Design review of the part shown in the three views and the two pictorial views. Dimensions are in mm from the part's minimum x, y and z. Round coordinates to 2 decimals unless told otherwise and drop trailing zeros. Write each loop counter-clockwise with the first axis right and the second up, starting at its lowest first coordinate (ties: lowest second). Pieces come first, ordered by that corner, then holes. Notation, with made-up numbers: (-2, 35) - (51, 35) arc R20 ccw to (51, 59) - close; hole circle Ø11 at (27, 39). An arc over 180 degrees is marked (long way). Use one line per item in the form item = value.
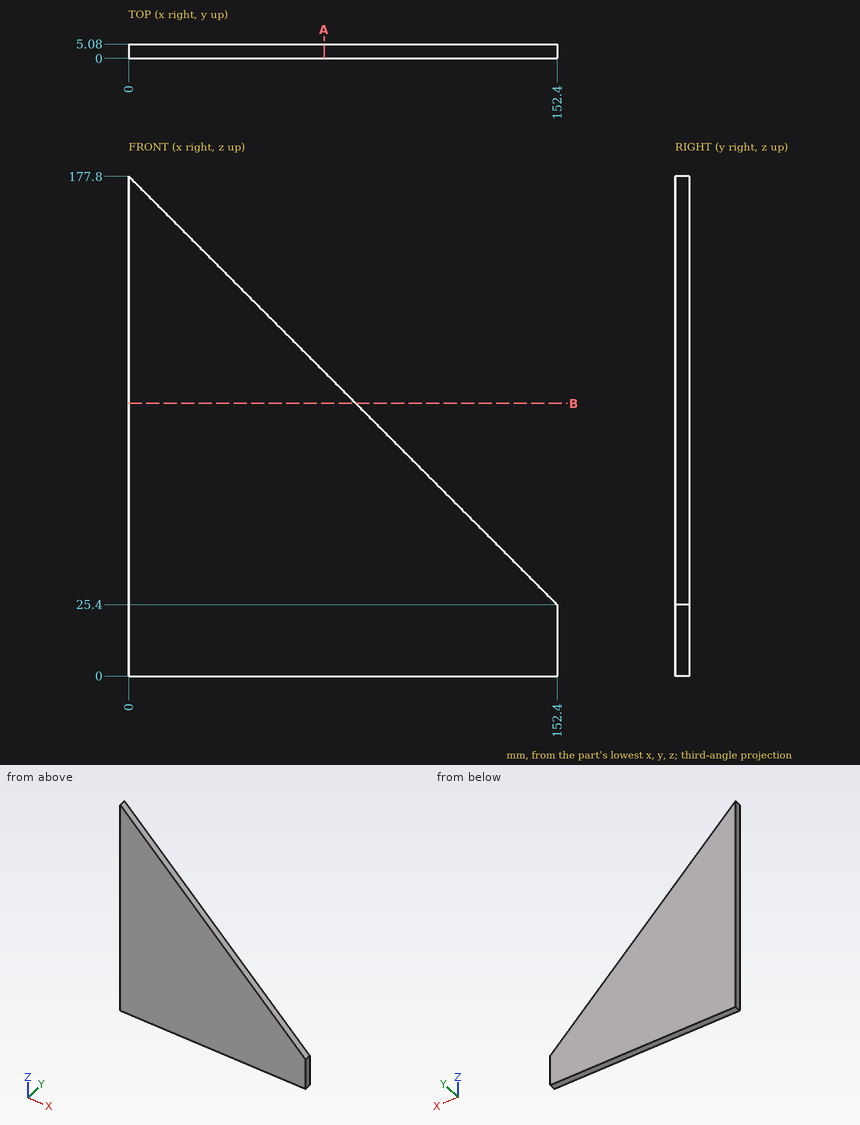
(1) Add section B-B on z = 97. Write out the cut boundary in (x, y), then the cut area to 3 significant figures.
Geometry results:
outline = (0, 0) - (80.8, 0) - (80.8, 5.08) - (0, 5.08) - close
area = 410 mm2
(2) To check wall thickness, follow L1, parallel to Z at x = 52.5, y = 4.1; L2, parallel to X at y = 1.5, z = 158; L3, parallel to X at y = 2.05, z = 47. State the ranges of each line that lie inside material, in increasing order.
Geometry results:
L1 = 0 to 125.3
L2 = 0 to 19.8
L3 = 0 to 130.8
(3) Add section A-A on x = 69.5. Write out the cut boundary in (y, z).
Geometry results:
outline = (0, 0) - (5.08, 0) - (5.08, 108.3) - (0, 108.3) - close
